The drawing under review shows one solid part. Ordinate dimensions are in mm from its lowest x, y, z. Give positions to 0.01 mm unless a question says otherwise; leave off trailing zeros. Loops run counter-clockwise (first coordinate to the right, second up) from the corner with the lowest first, then second, coordinate; pieces in that order, holes last. Notation, with made-up numbers: (34.5, 51.25) -> (87.5, 51.25) arc R6 ccw to (87.5, 62.25) -> close; hole circle Ø2 at (-19, -4.5). An arc over 180 degrees is marked (long way). Answer in a Markdown table with one row per item. Add a question column.
(1) For line 1 (X direction, y = 59, z = 2.4) (1 decimal); line 2 (X direction, y = 59.5, z = 1.45) (1 decimal); line 3 (X direction, y = 37.5, z = 1.4) (1 decimal), list the stretches that pass through material, from the lowest coordinate up.
(2) Consider section D-D on x = 62.5. Write out the cut boundary in (y, z) (1 decimal).
(3) For pin 1 (2 mm diameter, centred on x = 36.51, y = 20.01, fed in from +Z) (1 decimal); pin 2 (1.7 mm diameter, centred on x = 36.51, y = 44.01, fed in from -Z), all flat-tipped, find the tip position at first contact; note any pin that passes through.
(4) Consider section B-B on x = 32.5. Write out the cut boundary in (y, z) (1 decimal).
(5) Consider section C-C on z = 0.7. Count the separate pieces of the cut face and the enclosed holes in it, then the cut area to 3 significant figures.
(6) Consider section A-A on y = 34. Write out the cut boundary in (x, z) (1 decimal), then the cut area to 3 significant figures.
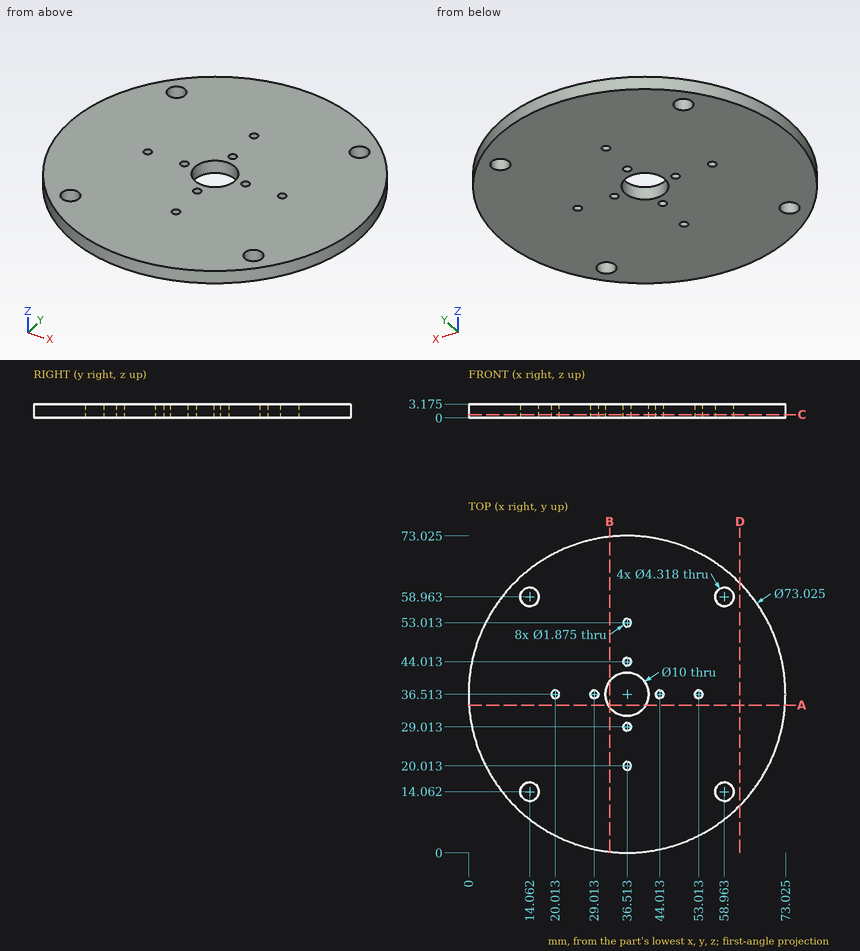
Values follow:
| question | item | result |
|---|---|---|
| 1 | line 1 | 7.7 to 11.9, 16.2 to 56.8, 61.1 to 65.3 |
| 1 | line 2 | 8.1 to 12, 16.2 to 56.9, 61.1 to 64.9 |
| 1 | line 3 | 0 to 31.6, 41.4 to 73 |
| 2 | outline | (10.9, 0) -> (62.2, 0) -> (62.2, 3.2) -> (10.9, 3.2) -> close |
| 3 | pin 1 | z = 3.2 |
| 3 | pin 2 | through |
| 4 | outline | (0.2, 0) -> (33.5, 0) -> (33.5, 3.2) -> (0.2, 3.2) -> close; (39.5, 0) -> (72.8, 0) -> (72.8, 3.2) -> (39.5, 3.2) -> close |
| 5 | separate pieces | 1 |
| 5 | enclosed holes | 13 |
| 5 | area | 4,030 mm2 |
| 6 | outline | (0.1, 0) -> (32.2, 0) -> (32.2, 3.2) -> (0.1, 3.2) -> close; (40.8, 0) -> (72.9, 0) -> (72.9, 3.2) -> (40.8, 3.2) -> close |
| 6 | area | 204 mm2 |
